Geometry check sheet. Reference: drawing and pictorial views, mm from the part's lowest x, y, z. Round coordinates to 2 decimals unless told otherwise and drop trailing zeros. Write each loop counter-clockwise with the first axis right and the second up, starting at its lowest first coordinate (ties: lowest second). Pieces come first, ordered by that corner, then holes. Notation, with made-up numbers: (46.25, 79.25) - (82.25, 79.25) arc R32 ccw to (82.25, 115.25) - close; hole circle Ø2 at (61.25, 5.25). An arc over 180 degrees is marked (long way). Use one line per item in the form item = value. Start each with the question number.
1) Gauge pin test, flat ends, axial feed: P1, Ø1, axis at y = 54.5, z = 1.5, coming from the +X side; P2, Ø0.6, axis at y = 87, z = 1.5, coming from the -X side; P3, Ø5.5, axis at x = 70, y = 65, coming from the +Z side. Record the tip position at first contact, or that the pin passes through.
2) Section check A-A (y = 65). Record the boundary of the cut face in (x, z).
3) Section check C-C (y = 20.5). Record the boundary of the cut face in (x, z).
4) Section check D-D (z = 1.3). Record the boundary of the cut face in (x, y).
5) Section check B-B (x = 35). Record the boundary of the cut face in (y, z).
6) Scan lines: probe 1 along Y at (x, z) = (70, 0.6); probe 2 along Y at (x, z) = (35, 1.65); probe 3 along X at (y, z) = (53, 1.45). Record each from-to range of solid material in increasing order.
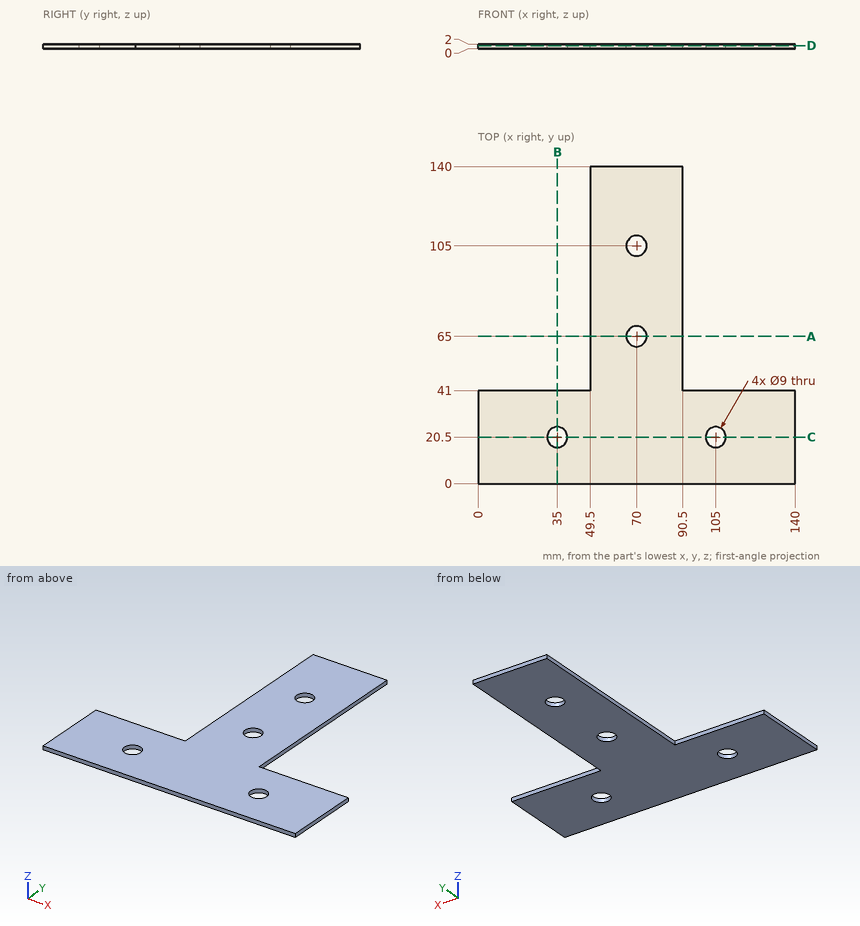
Results are:
q1.P1 = 90.5
q1.P2 = 49.5
q1.P3 = through
q2.outline = (49.5, 0) - (65.5, 0) - (65.5, 2) - (49.5, 2) - close; (74.5, 0) - (90.5, 0) - (90.5, 2) - (74.5, 2) - close
q3.outline = (0, 0) - (30.5, 0) - (30.5, 2) - (0, 2) - close; (39.5, 0) - (100.5, 0) - (100.5, 2) - (39.5, 2) - close; (109.5, 0) - (140, 0) - (140, 2) - (109.5, 2) - close
q4.outline = (0, 0) - (140, 0) - (140, 41) - (90.5, 41) - (90.5, 140) - (49.5, 140) - (49.5, 41) - (0, 41) - close; hole circle Ø9 at (35, 20.5); hole circle Ø9 at (70, 65); hole circle Ø9 at (70, 105); hole circle Ø9 at (105, 20.5)
q5.outline = (0, 0) - (16, 0) - (16, 2) - (0, 2) - close; (25, 0) - (41, 0) - (41, 2) - (25, 2) - close
q6.probe_1 = 0 to 60.5, 69.5 to 100.5, 109.5 to 140
q6.probe_2 = 0 to 16, 25 to 41
q6.probe_3 = 49.5 to 90.5
